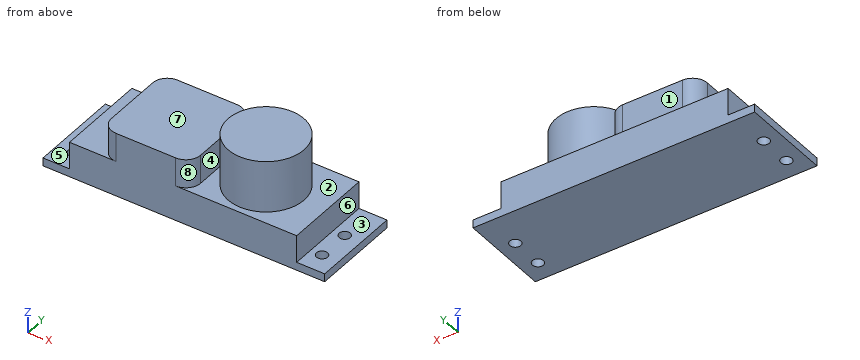
```python
from build123d import *

# Parameters (mm, degrees)
F0_W     = 38.2
F0_H     = 12.25
F0_R     = 0.75
F1_DEPTH = 1.1
F2_W     = 30.8
F2_H     = 12.25
F3_DEPTH = 3.7
F5_DEPTH = 3.9
F4_R     = 5.15
F6_DEPTH = 7


with BuildPart() as f1:
    # F0 (on Top) → F1 (new body)
    with BuildSketch(Plane.XY):
        Rectangle(F0_W, F0_H)
        with Locations((-16.85, -3.375)):
            Circle(F0_R, mode=Mode.SUBTRACT)
        with Locations((16.85, -3.375)):
            Circle(F0_R, mode=Mode.SUBTRACT)
        with Locations((-16.85, 1.075)):
            Circle(F0_R, mode=Mode.SUBTRACT)
        with Locations((16.85, 1.075)):
            Circle(F0_R, mode=Mode.SUBTRACT)
    extrude(amount=F1_DEPTH)

    # F2 (on face) → F3 (join)
    with BuildSketch(Plane.XY.offset(1.1)):
        with Locations((-0.1, 0)):
            Rectangle(F2_W, F2_H)
    extrude(amount=F3_DEPTH)

    # F4 (on face) → F5 (join)
    with BuildSketch(Plane.XY.offset(4.8)):
        with BuildLine():
            Line((-1.1, 5.975), (-9.2, 5.975))
            ThreePointArc((-9.2, 5.975), (-10.614214, 5.389214), (-11.2, 3.975))
            Line((-11.2, 3.975), (-11.2, -4.125))
            ThreePointArc((-11.2, -4.125), (-10.614214, -5.539214), (-9.2, -6.125))
            Line((-9.2, -6.125), (-1.1, -6.125))
            ThreePointArc((-1.1, -6.125), (0.314214, -5.539214), (0.9, -4.125))
            Line((0.9, -4.125), (0.9, 3.975))
            ThreePointArc((0.9, 3.975), (0.314214, 5.389214), (-1.1, 5.975))
        make_face()
    extrude(amount=F5_DEPTH)

    # F4 (on face) → F6 (join)
    with BuildSketch(Plane.XY.offset(4.8)):
        with Locations((7.05, -0.175)):
            Circle(F4_R)
    extrude(amount=F6_DEPTH)


solid = f1.part
```
Design review of the part built by this model. Coordinates are the model's own, in mm. Face numbers are marked on the shaded views. A direction names the side the tool comes from. Round coordinates to 2 decimals unless told otherwise and drop trailing zeros. Write each loop counter-clockwise with the first axis right and the second up, starting at its lowest first coordinate (ties: lowest second). Pieces come first, ordered by that corner, then holes. Notation, with made-up numbers: (84, 41.5) -> (118, 41.5) arc R29 cw to (118, 77.5) -> close; hole circle Ø5 at (-23, 78). An arc over 180 degrees is marked (long way). Write item = value, one per line. Start each with the question number.
1) Take a section at A-A, the plane x = 16.85. State the section outline as (y, z) points (3 decimals).
2) Wall thickness on probe 1 along Y at (x, z) = (-16.85, 0.55) (3 decimals); probe 2 along Z at (x, y) = (-5.5, 1.25); probe 3 along X at (y, z) = (0.75, 4.25): over which ranges is each line inside the solid? List them lowest first. Write a range as from..to.
3) Tool access review of the marked faces 1, 2, 3, 4 and 5: name each direction out of +Z, -Z, +X, -X, +Y, -Y from which nothing blocks a thin tool from reaching the whole face with its end or side.
4) Mouldability with a two-part tool opening along X and no side actions: class the marked faces 6, 7 and 8 as +X half, -X half, draft (parallel to the pull), parting line (faces both ways), or undercut.
5) Take a section at D-D, the plane z = 2.5. State the section outline as (x, y) points (3 decimals).
6) Take a section at C-C, the plane x = 7.05. State the section outline as (y, z) points (3 decimals).
7) Clearance check with flat-ended pins moving along their axes: pin 1 (3.5 mm diameter, centred on x = -2, y = 2.5, fed in from +Z); pin 2 (4 mm diameter, centred on x = -18, y = 0, fed in from +Z); pin 3 (6 mm diameter, centred on x = -1.5, z = 8.5, fed in from +Y) (3 decimals). State where each tip first meets the part, or that it passes through.
8) Take a section at B-B, the plane z = 5.5. State the section outline as (x, y) points (3 decimals), plus the area to 3 significant figures.
Results list:
q1.outline = (-6.125, 0) -> (-4.125, 0) -> (-4.125, 1.1) -> (-6.125, 1.1) -> close; (-2.625, 0) -> (0.325, 0) -> (0.325, 1.1) -> (-2.625, 1.1) -> close; (1.825, 0) -> (6.125, 0) -> (6.125, 1.1) -> (1.825, 1.1) -> close
q2.probe_1 = -6.125..-4.125, -2.625..0.325, 1.825..6.125
q2.probe_2 = 0..8.7
q2.probe_3 = -15.5..15.3
q3.face_1 = +Z, +X, -X, +Y
q3.face_2 = +Z
q3.face_3 = +Z, +X, +Y, -Y
q3.face_4 = +Z, +Y, -Y
q3.face_5 = +Z, -X, +Y, -Y
q4.face_6 = +X half
q4.face_7 = draft
q4.face_8 = undercut
q5.outline = (-15.5, -6.125) -> (15.3, -6.125) -> (15.3, 6.125) -> (-15.5, 6.125) -> close
q6.outline = (-6.125, 0) -> (6.125, 0) -> (6.125, 4.8) -> (4.975, 4.8) -> (4.975, 11.8) -> (-5.325, 11.8) -> (-5.325, 4.8) -> (-6.125, 4.8) -> close
q7.pin_1 = 8.7
q7.pin_2 = 1.1
q7.pin_3 = 5.975
q8.outline = (-11.2, -4.125) arc R2 ccw to (-9.2, -6.125) -> (-1.1, -6.125) arc R2 ccw to (0.9, -4.125) -> (0.9, 3.975) arc R2 ccw to (-1.1, 5.975) -> (-9.2, 5.975) arc R2 ccw to (-11.2, 3.975) -> close; circle Ø10.3 at (7.05, -0.175)
q8.area = 226 mm²
